For this review, use the dimensioned drawing (mm, ordinates from the lowest corner) and the shaded views. Round coordinates to 2 decimals unless told otherwise and drop trailing zeros. Write each loop counter-clockwise with the first axis right and the second up, starting at its lowest first coordinate (ties: lowest second). Pieces come first, ordered by that corner, then holes. Notation, with made-up numbers: M 67,12.25 L 98,12.25 A7 cw 98,25.25 Z; hole C -18,83 d2. An arc over 180 degrees is marked long. Use one line per item in the form item = value. Start each with the question number.
Item 1: Add section C-C (y = 47). State the section outline as (x, z) points, and give its area (3 significant figures).
Item 2: Add section A-A (y = 4.5). State the section outline as (x, z) points, and give its area (3 significant figures).
Item 3: For line 1 (X direction, y = 51.5, z = 15); line 2 (Y direction, x = 15, z = 6); line 3 (Z direction, x = 23, y = 53.5), list the stretches that pass through material, from the lowest coordinate up. Write a range as [from, to].
Item 4: Draft analysis for pull direction Z (two halves, no side actions). For the marked faces 1, 2, 3 and 4, state which applies: released by +Z, released by -Z, zero draft, split by the parting line, or undercut.
Item 5: For P1, Ø1.2, axis at x = 15.5, y = 47, coming from the +Z side; P2, Ø1.2, axis at x = 14.5, y = 11, coming from the -Z side; P3, Ø1.2, axis at x = 7.5, z = 15, coming from the +Y side, all flat-tipped, find the tip position at first contact; note any pin that passes through.
Item 6: Add section B-B (z = 15). State the section outline as (x, y) points, and give its area (3 significant figures).
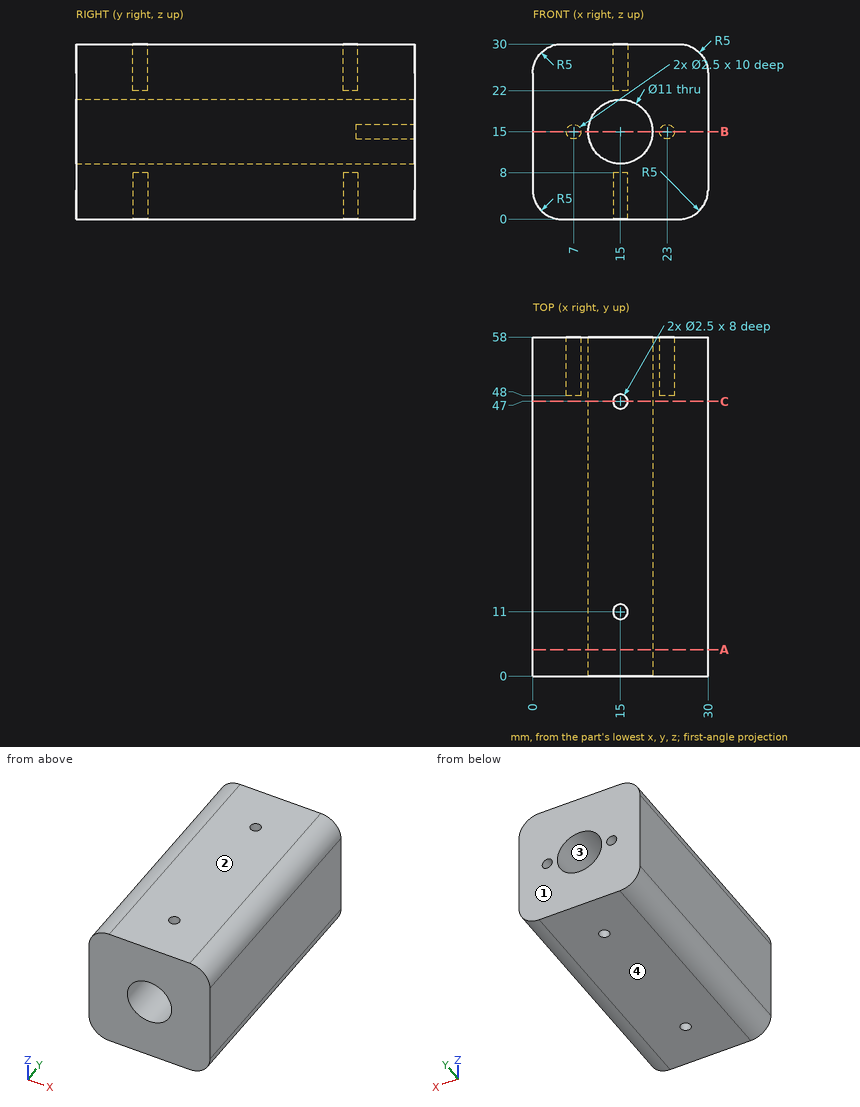
Calculated:
q1.outline = M 0,5 A5 ccw 5,0 L 13.75,0 L 13.75,8 L 16.25,8 L 16.25,0 L 25,0 A5 ccw 30,5 L 30,25 A5 ccw 25,30 L 16.25,30 L 16.25,22 L 13.75,22 L 13.75,30 L 5,30 A5 ccw 0,25 Z; hole C 15,15 d11
q1.area = 744 mm^2
q2.outline = M 0,5 A5 ccw 5,0 L 25,0 A5 ccw 30,5 L 30,25 A5 ccw 25,30 L 5,30 A5 ccw 0,25 Z; hole C 15,15 d11
q2.area = 784 mm^2
q3.line_1 = [0, 5.75], [8.25, 9.5], [20.5, 21.75], [24.25, 30]
q3.line_2 = [0, 9.75], [12.25, 45.75], [48.25, 58]
q3.line_3 = [0, 13.75], [16.25, 30]
q4.face_1 = zero draft
q4.face_2 = released by +Z
q4.face_3 = undercut
q4.face_4 = released by -Z
q5.P1 = 22
q5.P2 = 8
q5.P3 = 48
q6.outline = M 0,0 L 9.5,0 L 9.5,58 L 8.25,58 L 8.25,48 L 5.75,48 L 5.75,58 L 0,58 Z; M 20.5,0 L 30,0 L 30,58 L 24.25,58 L 24.25,48 L 21.75,48 L 21.75,58 L 20.5,58 Z
q6.area = 1,050 mm^2
